Could you check a few things on this drawing? It's one solid part, dimensions in mm from its lowest x, y, z. A direction names the side the tool comes from. Coordinates: 2 decimals unless noted, no trailing zeros. Order: outer loops, then holes, each group sorted by start corner. A loop starts at its lowest first (then second) coordinate and runs counter-clockwise, first axis right, second up.
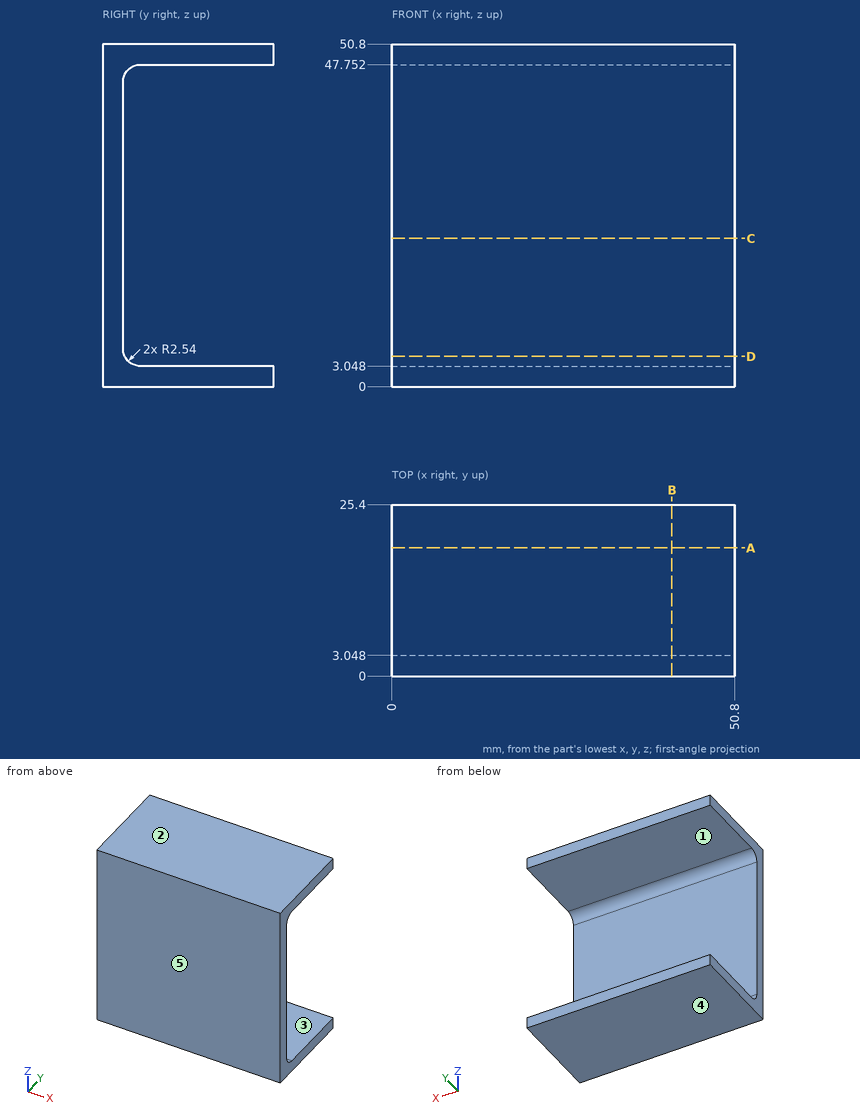
1. Please list where these lines run through material, in increasing order: probe 1 along Z at (x, y) = (19, 5.75); probe 2 along Y at (x, z) = (24, 32.5); probe 3 along Z at (x, y) = (48.5, 4.5).
Completed:
probe 1: z = 0 to 3.05, 47.75 to 50.8
probe 2: y = 0 to 3.05
probe 3: z = 0 to 3.29, 47.51 to 50.8
2. Imagine slicing it at A-A on y = 19. Please give me the cut outline in (x, z).
Completed:
outline: (0, 0) - (50.8, 0) - (50.8, 3.05) - (0, 3.05) - close; (0, 47.75) - (50.8, 47.75) - (50.8, 50.8) - (0, 50.8) - close
3. Imagine slicing it at B-B on x = 41.5. Please give me the cut outline in (y, z), then the cut area to 3 significant figures.
Completed:
outline: (0, 0) - (25.4, 0) - (25.4, 3.05) - (5.59, 3.05) arc R2.54 cw to (3.05, 5.59) - (3.05, 45.21) arc R2.54 cw to (5.59, 47.75) - (25.4, 47.75) - (25.4, 50.8) - (0, 50.8) - close
area: 294 mm2
4. Imagine slicing it at C-C on z = 22. Please give me the cut outline in (x, y), then the cut area to 3 significant figures.
Completed:
outline: (0, 0) - (50.8, 0) - (50.8, 3.05) - (0, 3.05) - close
area: 155 mm2
5. On a 3-axis mill with a long thin cutter (end or side, diameter ignored), from which of +Z, -Z, +X, -X, +Y, -Y can I reach the whole of each face in a straight line? I mean the marked faces 1 and 2. Say none if no direction works.
Completed:
face 1: +X, -X, +Y
face 2: +Z, +X, -X, +Y, -Y
6. Imagine slicing it at D-D on z = 4.5. Please give me the cut outline in (x, y), then the cut area to 3 significant figures.
Completed:
outline: (0, 0) - (50.8, 0) - (50.8, 3.29) - (0, 3.29) - close
area: 167 mm2
7. Thinking about a two-plate mould opening in Z: for the marked faces 3, 4 and 5, which applies, pulls with the +Z half, pulls with the -Z half, needs draft (parallel to the pull), parting line crosses it, or undercut?
Completed:
face 3: undercut
face 4: pulls with the -Z half
face 5: needs draft
8. I'm going to push a flat-ended pin straight in: pin 1 (4 mm diameter, centred on x = 16, z = 9, fed in from +Y). Where does the tip first touch, or does it pass through?
Completed:
pin 1: stops at y = 3.05
